Job drawing, mm, ordinate dimensions from the low corner. One solid piece. A direction names the side the tool comes from. Give positions to 0.01 mm unless a question says otherwise; leave off trailing zeros. Loops run counter-clockwise (first coordinate to the right, second up) from the corner with the lowest first, then second, coordinate; pieces in that order, holes last.
Item 1: Saw through at C-C on x = 63. Give the cut face in (y, z).
Item 2: Drop flat-ended pins along their axis: P1, Ø3, axis at x = 75.5, y = 9, coming from the +Z side; P2, Ø4, axis at x = 31.5, y = 15.5, coming from the -Z side; P3, Ø5, axis at y = 17.5, z = 17, coming from the +X side. Give the stop position or say it passes through.
Item 3: Probe probe 1 along Z at (x, y) = (67, 8.5); probe 2 along X at (y, z) = (3, 16.5); probe 3 along X at (y, z) = (17.5, 5.25) (1 decimal). List the from-to ranges inside material, lowest first.
Item 4: Saw through at B-B on z = 3.5. Give the cut face in (x, y).
Item 5: Saw through at D-D on y = 17. Give the cut face in (x, z).
Item 6: Which spindle directions (+Z, -Z, +X, -X, +Y, -Y) get a long thin tool onto all of the face, cutting with end or side? Do the marked faces 1, 2 and 3. Say none if no direction does.
Item 7: Saw through at A-A on y = 22.75. Give the cut face in (x, z).
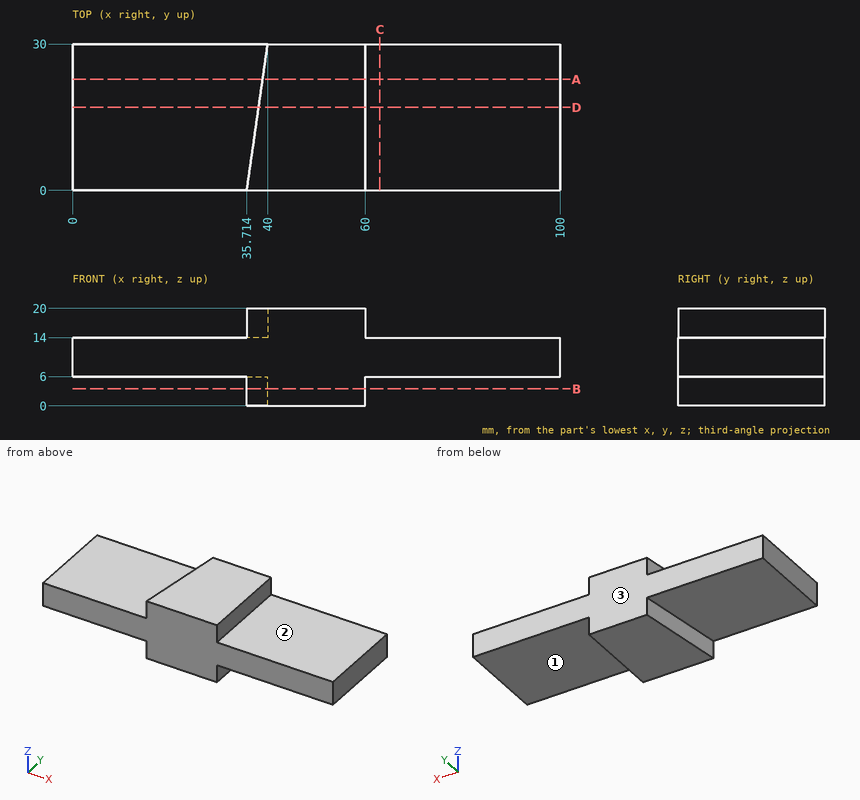
Results below:
1. outline: (0, 6) - (30, 6) - (30, 14) - (0, 14) - close
2. P1: stops at z = 14
2. P2: stops at z = 6
2. P3: stops at x = 60
3. probe 1: z = 6 to 14
3. probe 2: x = 36.14 to 60
3. probe 3: x = 38.2 to 60
4. outline: (35.71, 0) - (60, 0) - (60, 30) - (40, 30) - close
5. outline: (0, 6) - (38.14, 6) - (38.14, 0) - (60, 0) - (60, 6) - (100, 6) - (100, 14) - (60, 14) - (60, 20) - (38.14, 20) - (38.14, 14) - (0, 14) - close
6. face 1: -Z, +X, +Y, -Y
6. face 2: +Z, +X, +Y, -Y
6. face 3: +Z, -Z, +X, -X, +Y
7. outline: (0, 6) - (38.96, 6) - (38.96, 0) - (60, 0) - (60, 6) - (100, 6) - (100, 14) - (60, 14) - (60, 20) - (38.96, 20) - (38.96, 14) - (0, 14) - close
